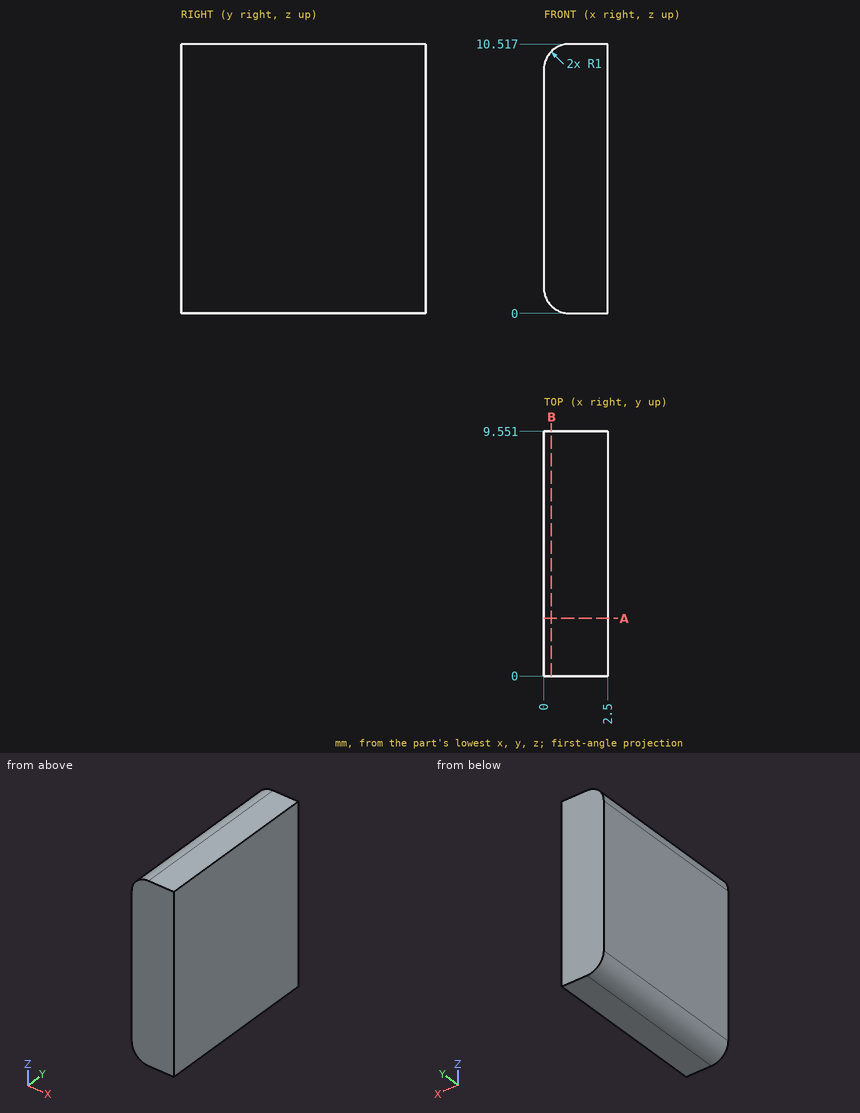
Job drawing, mm, ordinate dimensions from the low corner. One solid piece. Give positions to 0.01 mm unless a question says otherwise; leave off trailing zeros. Write each loop counter-clockwise with the first axis right and the second up, starting at its lowest first coordinate (ties: lowest second). Pieces come first, ordered by that corner, then holes. Notation, with made-up numbers: M 40.25,50 L 51.25,50 A25 ccw 51.25,89 Z; hole C -7,38 d10. An arc over 180 degrees is marked long. One line per item, written item: value. Start each with the question number.
Q1. Saw through at B-B, the plane x = 0.3. Write the cut outline in (y, z).
Q2. Saw through at A-A, the plane y = 2.25. Write the cut outline in (x, z).
Q3. Probe probe 1 along Z at (x, y) = (0.95, 5); probe 2 along Z at (x, y) = (0.3, 1.75). List the from-to ranges inside material, lowest first. Write a range as [from, to].
Q4. Drop a flat-ended pin along its axis: pin 1 Ø1 at (x, z) = (1.5, 2.5) entering from -Y. Give the stop position or say it passes through.
Output values:
1. outline: M 0,0.29 L 9.55,0.29 L 9.55,10.23 L 0,10.23 Z
2. outline: M 0,1 A1 ccw 1,0 L 2.5,0 L 2.5,10.52 L 1,10.52 A1 ccw 0,9.52 Z
3. probe 1: z = [0, 10.52]
3. probe 2: z = [0.29, 10.23]
4. pin 1: stops at y = 0
